from build123d import *

# Parameters (mm, degrees)
CROQUIS1_R              = 1.5
SALIENTE_EXTRUIR1_DEPTH = 2.5


with BuildPart() as part:
    # Croquis1 → Saliente-Extruir1 (new body)
    with BuildSketch(Plane.XY):
        with BuildLine():
            Line((-5, 36.080727307), (-5, 0))
            ThreePointArc((-5, 0), (0, -5), (5, 0))
            Line((5, 0), (5, 51.928629296))
            Line((5, 51.928629296), (2.885723707, 53.262734147))
            Line((2.885723707, 53.262734147), (-5, 40.765516506))
            Line((-5, 40.765516506), (-2.885723707, 39.431411654))
            Line((-2.885723707, 39.431411654), (-5, 36.080727307))
        make_face()
        Circle(CROQUIS1_R, mode=Mode.SUBTRACT)
        with Locations((0, 30)):
            Circle(CROQUIS1_R, mode=Mode.SUBTRACT)
    extrude(amount=SALIENTE_EXTRUIR1_DEPTH)


solid = part.part
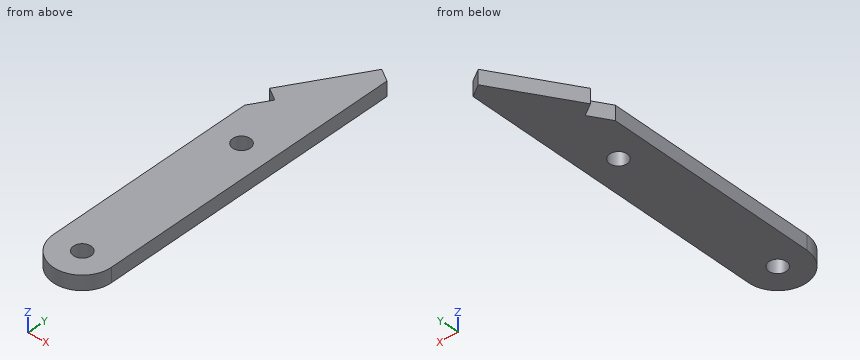
Could you check a few things on this model? Use its own coordinates, in mm. Give positions to 0.01 mm unless a question says otherwise; leave off trailing zeros. Loops run counter-clockwise (first coordinate to the right, second up) from the corner with the lowest first, then second, coordinate; pieces in that order, holes last. Notation, with made-up numbers: (-6, -29) -> (19, -29) arc R21 ccw to (19, -16) -> close; hole circle Ø3 at (33, 39.25). An arc over 180 degrees is marked (long way). Return JSON: item names as keys, results as strings.
Item 1: I'm going to push flat-ended pins straight in: pin 1 (1.5 mm diameter, centred on x = 2.5, z = 0.5, fed in from -Y); pin 2 (2.5 mm diameter, centred on x = 0, y = 0, fed in from +Z). Where does each tip first touch, or does it pass through?
Geometry results:
{"pin 1": "stops at y = -4.68", "pin 2": "passes through"}
Item 2: If we section it at C-C on x = 1: List the corners of the cut face in (y, z) for me.
Geometry results:
{"outline": "(-4.9, 0) -> (-1.12, 0) -> (-1.12, 2.5) -> (-4.9, 2.5) -> close; (1.12, 0) -> (28.88, 0) -> (28.88, 2.5) -> (1.12, 2.5) -> close; (31.12, 0) -> (50.27, 0) -> (50.27, 2.5) -> (31.12, 2.5) -> close"}
Item 3: If we section it at B-B on z = 0.6: List the corners of the cut face in (x, y) for me, plus the area to 3 significant figures.
Geometry results:
{"outline": "(-5, 0) arc R5 ccw to (5, 0) -> (5, 51.93) -> (2.89, 53.26) -> (-5, 40.77) -> (-2.89, 39.43) -> (-5, 36.08) -> close; hole circle Ø3 at (0, 0); hole circle Ø3 at (0, 30)", "area": "502 mm²"}
Item 4: If we section it at A-A on y = 30: List the corners of the cut face in (x, z) for me, plus the area to 3 significant figures.
Geometry results:
{"outline": "(-5, 0) -> (-1.5, 0) -> (-1.5, 2.5) -> (-5, 2.5) -> close; (1.5, 0) -> (5, 0) -> (5, 2.5) -> (1.5, 2.5) -> close", "area": "17.5 mm²"}
Item 5: If we section it at D-D on x = -4: List the corners of the cut face in (y, z) for me, plus the area to 3 significant figures.
Geometry results:
{"outline": "(-3, 0) -> (37.67, 0) -> (37.67, 2.5) -> (-3, 2.5) -> close; (40.13, 0) -> (42.35, 0) -> (42.35, 2.5) -> (40.13, 2.5) -> close", "area": "107 mm²"}
Item 6: I need wall thicknesses on L1, parallel to Y at x = 0, z = 1.95; L2, parallel to Y at x = -1, z = 2.3; L3, parallel to Y at x = -3.25, z = 1.2. Which ranges of each line are inside material? Lowest first, please. Write a range as from..to.
Geometry results:
{"L1": "y = -5..-1.5, 1.5..28.5, 31.5..48.69", "L2": "y = -4.9..-1.12, 1.12..28.88, 31.12..47.1", "L3": "y = -3.8..38.85, 39.66..43.54"}
